Check sheet for the drawn part. Datum: minimum x, y, z corner. Units: mm. A direction names the side the tool comes from. Coordinates: 2 decimals unless noted, no trailing zeros. Write each loop counter-clockwise with the first axis right and the second up, starting at its lowest first coordinate (ties: lowest second). Pieces come first, ordered by that corner, then holes. Notation, with made-up numbers: (11.5, 78) - (53.5, 78) arc R20 cw to (53.5, 107) - close; hole circle Ø6 at (52, 74.25). An arc over 180 degrees is marked (long way). Use CSV: the item, a comma, the result in double quotes. Start each with the question number.
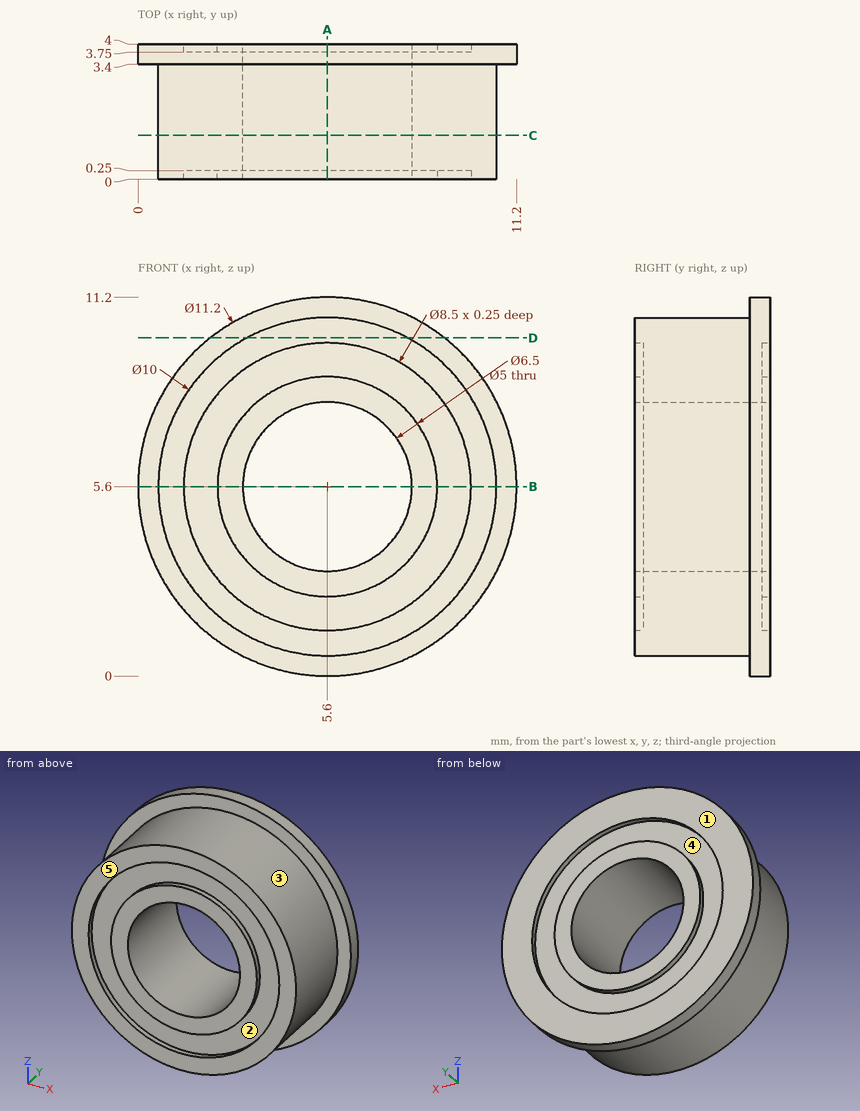
Q1. Cross-section at B-B (z = 5.6). Record the cut outline in (x, y), plus the area to 3 significant figures.
Q2. Gauge pin test, flat end, axial feed: pin 1 (1 mm diameter, centred on x = 4.5, y = 2, fed in from +Z). Record the tip position at first contact, or that the pin passes through.
Q3. Release check for a two-part mould opening along X. For the marked faces 3, 4 and 5 record: released by +X, released by -X, zero draft, split by the parting line, or undercut.
Q4. Scan lines: line 1 along Z through (x, y) = (5.6, 2.6); line 2 along Z through (x, y) = (5, 1.1); line 3 along Y through (x, z) = (4, 2.5). Record each from-to range of solid material in increasing order. Write a range as from..to.
Q5. Cross-section at C-C (y = 1.3). Record the cut outline in (x, z).
Q6. Cross-section at A-A (x = 5.6). Record the cut outline in (y, z).
Q7. Tool access check on the marked faces 1 and 2. Record the directions out of +Z, -Z, +X, -X, +Y, -Y that give a thin tool (end or side, any length) a straight path to the whole face; none if there is none.
Q8. Cross-section at D-D (z = 10). Record the cut outline in (x, y).
Reply:
1,outline,"(0, 3.4) - (0.6, 3.4) - (0.6, 0) - (1.35, 0) - (1.35, 0.25) - (2.35, 0.25) - (2.35, 0) - (3.1, 0) - (3.1, 4) - (2.35, 4) - (2.35, 3.75) - (1.35, 3.75) - (1.35, 4) - (0, 4) - close; (8.1, 0) - (8.85, 0) - (8.85, 0.25) - (9.85, 0.25) - (9.85, 0) - (10.6, 0) - (10.6, 3.4) - (11.2, 3.4) - (11.2, 4) - (9.85, 4) - (9.85, 3.75) - (8.85, 3.75) - (8.85, 4) - (8.1, 4) - close"
1,area,"19.7 mm^2"
2,pin 1,"z = 10.56"
3,face 3,"split by the parting line"
3,face 4,"undercut"
3,face 5,"zero draft"
4,line 1,"0.6..3.1, 8.1..10.6"
4,line 2,"0.64..3.17, 8.03..10.56"
4,line 3,"0.25..3.75"
5,outline,"circle Ø10 at (5.6, 5.6); hole circle Ø5 at (5.6, 5.6)"
6,outline,"(0, 0.6) - (3.4, 0.6) - (3.4, 0) - (4, 0) - (4, 1.35) - (3.75, 1.35) - (3.75, 2.35) - (4, 2.35) - (4, 3.1) - (0, 3.1) - (0, 2.35) - (0.25, 2.35) - (0.25, 1.35) - (0, 1.35) - close; (0, 8.1) - (4, 8.1) - (4, 8.85) - (3.75, 8.85) - (3.75, 9.85) - (4, 9.85) - (4, 11.2) - (3.4, 11.2) - (3.4, 10.6) - (0, 10.6) - (0, 9.85) - (0.25, 9.85) - (0.25, 8.85) - (0, 8.85) - close"
7,face 1,"+Z, -Z, +X, -X, +Y"
7,face 2,"-Y"
8,outline,"(2.14, 3.4) - (3.23, 3.4) - (3.23, 0) - (7.97, 0) - (7.97, 3.4) - (9.06, 3.4) - (9.06, 4) - (2.14, 4) - close"
